Autodesk Fusion 360 part; units mm, degrees
sketch "Skectch1" plane through (0, 0, 0) normal (0, 0, 1) x (1, 0, 0)
  line L0 (0, 0) -> (63.9, 0)
  line L1 (63.9, 0) -> (63.9, 64.4)
  line L2 (63.9, 64.4) -> (0, 64.4)
  line L3 (0, 64.4) -> (0, 0)
  line L4 (-9.5, 73.9) -> (73.4, 73.9)
  line L5 (73.4, 73.9) -> (73.4, -9.5)
  line L6 (73.4, -9.5) -> (-9.5, -9.5)
  line L7 (-9.5, -9.5) -> (-9.5, 73.9)
  circle A0 centre (-4.5, -4.5) radius 1.7
  circle A1 centre (68.4, -4.5) radius 1.7
  circle A2 centre (68.4, 68.9) radius 1.7
  circle A3 centre (-4.5, 68.9) radius 1.7
  circle A4 centre (-4.5, -4.5) radius 3
  circle A5 centre (68.4, -4.5) radius 3
  circle A6 centre (68.4, 68.9) radius 3
  circle A7 centre (-4.5, 68.9) radius 3
  dimension "d1" = 63.9
  dimension "d2" = 64.4
  dimension "d3" = 82.9
  dimension "d4" = 83.4
  dimension "d6" = 9.5
  dimension "d7" = 3.4
  dimension "d8" = 5
  dimension "d9" = 5
  dimension "d10" = 3.4
  dimension "d11" = 5
  dimension "d12" = 5
  dimension "d13" = 3.4
  dimension "d14" = 5
  dimension "d15" = 5
  dimension "d16" = 9.5
  dimension "d17" = 3.4
  dimension "d18" = 5
  dimension "d19" = 5
  dimension "d21" = 6
  dimension "d22" = 6
  dimension "d23" = 6
  dimension "d24" = 6
extrude "Extrude1" add sketch "Skectch1" along normal blind 9.9 from surface at 3.1 contours A4 | A5 | A6 | A7 makes body 1 at (70.9599, 70.4643, 9.7) makes body 2 at (-1.6809, 67.8739, 9.7) makes body 3 at (69.2125, -1.6121, 9.7) makes body 4 at (-1.5037, -4.6495, 9.7)
extrude "Extrude2" add sketch "Skectch1" along normal blind 13 contours L4 L5 L6 L7 bodies 1 2 3 4
extrude "Extrude3" add sketch "Skectch1" along normal blind 3 contours L0 L1 L2 L3 bodies 1
sketch "Sketch3" plane through (0, 0, 13) normal (0, 0, 1) x (-1, 0, 0)
  circle A0 centre (-68.4, -68.9) radius 1.7
  circle A1 centre (4.5, 4.5) radius 1.7
  line L0 (0, 0) -> (0, -64.4)
  line L1 (0, -64.4) -> (-63.9, -64.4)
  line L2 (-63.9, -64.4) -> (-63.9, 0)
  line L3 (-63.9, 0) -> (0, 0)
  line L4 (9.5, 9.5) -> (-73.4, 9.5)
  line L5 (-73.4, 9.5) -> (-73.4, -73.9)
  line L6 (-73.4, -73.9) -> (9.5, -73.9)
  line L7 (9.5, -73.9) -> (9.5, 9.5)
  circle A2 centre (4.5, -68.9) radius 1.7
  circle A3 centre (-68.4, 4.5) radius 1.7
  line L8 (-23.35, -73.9) -> (-41.85, -73.9)
  line L9 (-41.85, -73.9) -> (-41.85, -64.4)
  line L10 (-41.85, -64.4) -> (-23.35, -64.4)
  line L11 (-23.35, -64.4) -> (-23.35, -73.9)
  line L12 (9.5, 9.5) -> (9.5, -73.9)
  line L13 (-73.4, -73.9) -> (-73.4, 9.5)
  dimension "d32" = 18.5
  dimension "d33" = 32.85
  dimension "d34" = 31.55
extrude "Extrude4" cut sketch "Sketch3" against normal blind 7.5 contours L1 L6 L8 L9 L10 L11 bodies 1
fillet "Fillet1" radius 5 4 edges at (73.4, -9.5, 6.5) (73.4, 73.9, 6.5) (-9.5, 73.9, 6.5) (-9.5, -9.5, 6.5) on bodies 1
Source: CAD feature listing. Evaluate the final solid. Frame: model axes, mm. A direction names the side the tool comes from. Round coordinates to 2 decimals unless told otherwise and drop trailing zeros. Write each loop counter-clockwise with the first axis right and the second up, starting at its lowest first coordinate (ties: lowest second). Pieces come first, ordered by that corner, then holes. Notation, with made-up numbers: (80.25, 53.25) - (117.25, 53.25) arc R22 ccw to (117.25, 72.25) - close; hole circle Ø2 at (-19.75, 12). An arc over 180 degrees is marked (long way). Use CSV: the item, a comma, the result in double quotes. Start each with the question number.
(1) Cut plane A-A, the plane z = 6.5. Return loops of the section in (x, y).
(2) Set-up query: faces 4 (the face through (0, 33, 8)), 5 (the face through (-3.116, -1.838, 1.528)), 6 (the face through (68.179, 67.214, 7.981)). Return all of +Z, -Z, +X, -X, +Y, -Y with unobstructed straight access to the full face (end or side cutting, diameter ignored); none if empty.
(3) Mould query, pull axis X, two halves, no side actions, for faces 1 (the face through (-9.5, 32, 6)), 2 (the face through (31, 33, 0)), 3 (the face through (-4.721, 67.214, 7.981)). Classes: pulls with the +X half, pulls with the -X half, needs draft (parallel to the pull), parting line crosses it, or undercut.
(4) Material intervals for probe 1 along Y at (x, z) = (-4.5, 1.9); probe 2 along Y at (x, z) = (68.4, 10); probe 3 along X at (y, z) = (4, 10.75), sorted ascending. Write a range as [from, to].
(5) Cut plane C-C, the plane x = 21.5. Return loops of the section in (y, z).
(6) Cut plane B-B, the plane y = 63. Return loops of the section in (x, z).
(7) First-contact query: pin 1 Ø2 at (x, y) = (22, 35) entering from +Z; pin 2 Ø4 at (x, y) = (-4.5, -4.5) entering from -Z; pin 3 Ø3 at (x, y) = (35.5, 69) entering from +Z; pin 4 Ø2 at (x, y) = (-4.5, 68.9) entering from -Z (1 decimal). Flat tips, straight axial feed; report the tip coordinate or a pass-through.
Geometry says:
1,outline,"(-9.5, -4.5) arc R5 ccw to (-4.5, -9.5) - (68.4, -9.5) arc R5 ccw to (73.4, -4.5) - (73.4, 68.9) arc R5 ccw to (68.4, 73.9) - (41.85, 73.9) - (41.85, 64.4) - (63.9, 64.4) - (63.9, 0) - (0, 0) - (0, 64.4) - (23.35, 64.4) - (23.35, 73.9) - (-4.5, 73.9) arc R5 ccw to (-9.5, 68.9) - close; hole circle Ø3.4 at (-4.5, -4.5); hole circle Ø3.4 at (-4.5, 68.9); hole circle Ø3.4 at (68.4, -4.5); hole circle Ø3.4 at (68.4, 68.9)"
2,face 4,"+Z"
2,face 5,"-Z"
2,face 6,"+Z, -Z"
3,face 1,"pulls with the -X half"
3,face 2,"needs draft"
3,face 3,"undercut"
4,probe 1,"[-9.5, -7.5], [-1.5, 65.9], [71.9, 73.9]"
4,probe 2,"[-9.5, -6.2], [-2.8, 67.2], [70.6, 73.9]"
4,probe 3,"[-9.5, 0], [63.9, 73.4]"
5,outline,"(-9.5, 0) - (73.9, 0) - (73.9, 13) - (64.4, 13) - (64.4, 3) - (0, 3) - (0, 13) - (-9.5, 13) - close"
6,outline,"(-9.5, 0) - (73.4, 0) - (73.4, 13) - (63.9, 13) - (63.9, 3) - (0, 3) - (0, 13) - (-9.5, 13) - close"
7,pin 1,"z = 3"
7,pin 2,"z = 3.1"
7,pin 3,"z = 5.5"
7,pin 4,"through"
